The model under review builds one solid part; all positions refer to its coordinate system, in mm. A direction names the side the tool comes from. Give positions to 0.01 mm unless a question says otherwise; leave off trailing zeros. Write each loop counter-clockwise with the first axis right and the second up, starting at its lowest first coordinate (ties: lowest second). Pieces come first, ordered by that corner, then holes.
Autodesk Inventor part; units mm, degrees
ref_plane "Płaszczyzna konstrukcyjna1" through (0, -12, 0) normal (0, 0, -1) x (-1, 0, 0)
ref_plane "Płaszczyzna konstrukcyjna2" through (0, -10, -2.2657) normal (1, 0, 0) x (0, 0, -1)
ref_plane "YZ Plane" through (0, 0, 0) normal (1, 0, 0) x (0, 1, 0)
sketch "Szkic1" plane through (0, 0, 0) normal (0, 1, 0) x (-1, 0, 0)
  circle A0 centre (0, 0) radius 12.5
  circle A1 centre (0, 0) radius 10
  dimension "d0" = 20
  dimension "d2" = 25
extrude "Wyciągnięcie proste1" add sketch "Szkic1" along normal blind 5
ref_plane "Płaszczyzna konstrukcyjna1" through (0, -12, 0) normal (0, 0, -1) x (-1, 0, 0)
sketch "Szkic5" plane through (0, -12, 0) normal (0, 0, -1) x (-1, 0, 0)
  line L0 (12.5, 17) -> (-12.5, 17)
  line L1 (0, 17) -> (-12.5, 17)
  line L2 (-12.5, 17) -> (-12.5, 18.625)
  line L3 (-12.5, 18.625) -> (0, 18.625)
  line L4 (0, 18.625) -> (0, 17)
  line L5 (0, 18.625) -> (-9.5, 18.625)
  line L6 (-9.5, 18.625) -> (-9.5, 21.125)
  line L7 (-9.5, 21.125) -> (0, 21.125)
  line L8 (0, 21.125) -> (0, 18.625)
  line L9 (0, 21.125) -> (-12.5, 21.125)
  line L10 (-12.5, 21.125) -> (-12.5, 22.75)
  line L11 (-12.5, 22.75) -> (0, 22.75)
  line L12 (0, 22.75) -> (0, 21.125)
  line L13 (0, 22.75) -> (-9.5, 22.75)
  line L14 (-9.5, 22.75) -> (-9.5, 25.25)
  line L15 (-9.5, 25.25) -> (0, 25.25)
  line L16 (0, 25.25) -> (0, 22.75)
  line L17 (0, 25.25) -> (-12.5, 25.25)
  line L18 (-12.5, 25.25) -> (-12.5, 26.875)
  line L19 (-12.5, 26.875) -> (0, 26.875)
  line L20 (0, 26.875) -> (0, 25.25)
  line L21 (0, 26.875) -> (-9.5, 26.875)
  line L22 (-9.5, 26.875) -> (-9.5, 29.375)
  line L23 (-9.5, 29.375) -> (0, 29.375)
  line L24 (0, 29.375) -> (0, 26.875)
  line L25 (0, 29.375) -> (-12.5, 29.375)
  line L26 (-12.5, 29.375) -> (-12.5, 31)
  line L27 (-12.5, 31) -> (0, 31)
  line L28 (0, 31) -> (0, 29.375)
  line L29 (-12.5, 12) -> (-12.5, 17) construction
  line L30 (-12.5, 12) -> (-12.5, 17) construction
  line L31 (-12.5, 12) -> (12.5, 12) construction
  point P0 (0, 12)
  dimension "d13" = 2.5
  dimension "d17" = 19
  dimension "d18" = 3
revolve "Obrót1" add sketch "Szkic5" angle 360 about axis through (0, 10.75, 0) along (0, -1, 0)
sketch "Szkic7" plane through (0, 17.375, 0) normal (0, -1, 0) x (1, 0, 0)
  circle A0 centre (0, 0) radius 9.5
  circle A1 centre (0, 9.5) radius 1.65
  circle A2 centre (0, 0) radius 10
  circle A3 centre (0, 0) radius 9.5
  circle A4 centre (-9.5, 0) radius 1.65
  circle A5 centre (0, -9.5) radius 1.65
  circle A6 centre (9.5, 0) radius 1.65
  circle A7 centre (6.7175, -6.7175) radius 0.9
  circle A8 centre (6.7175, 6.7175) radius 0.9
  circle A9 centre (-6.7175, 6.7175) radius 0.9
  circle A10 centre (-6.7175, -6.7175) radius 0.9
  line L0 (6.7175, 6.7175) -> (0, 0) construction
  line L1 (0, 0) -> (-6.7175, 6.7175) construction
  circle A11 centre (0, 0) radius 12.5 construction
  line L2 (0, 0) -> (-6.7175, -6.7175) construction
  line L3 (0, 0) -> (6.7175, -6.7175) construction
  line L4 (17.5, 0) -> (-17.5, 0) construction
  dimension "d23" = 45
  dimension "d24" = 45
  dimension "d25" = 3.3
  dimension "d47" = 1.8
extrude "Wyciągnięcie proste6" cut sketch "Szkic7" along normal up to surface (10.75 mm away) contours A0 A6 | A0 A6 A2 | A8 A0 | A0 A8 A2 | A6 A2 | A7 A2 A0 | A0 A7 | A2 A8 | A7 A2 | A1 A0 | A0 A1 A2 | A5 A2 A0 | A0 A5 | A2 A1 | A5 A2 | A9 A0 | A0 A9 A2 | A10 A2 A0 | A0 A10 | A2 A9 | A10 A2 | A4 A0 | A0 A4 A2 | A2 A4
sketch "Szkic8" plane through (0, -12, 0) normal (0, 0, -1) x (-1, 0, 0)
  line L0 (6.0517, 25.25) -> (1.6438, 25.25)
  line L1 (-1.6438, 25.25) -> (-1.6438, 22.75)
  line L2 (1.6438, 25.25) -> (-1.6438, 25.25)
  line L3 (-1.6438, 25.25) -> (-1.6438, 22.75)
  line L4 (-1.6438, 22.75) -> (1.6438, 22.75)
  line L5 (1.6438, 22.75) -> (1.6438, 25.25)
  point P0 (0, 12)
  point P1 (1.65, 22.75)
extrude "Wyciągnięcie proste7" cut sketch "Szkic8" along normal through all both and the other way through all
sketch "Szkic9" plane through (0, 5, 0) normal (0, -1, 0) x (1, 0, 0)
  line L0 (0, 0) -> (-3.4352, 0)
  line L1 (-3.4352, 0) -> (-3.4352, -2.2657)
  line L2 (-3.4352, -2.2657) -> (0, -2.2657)
  line L3 (0, -2.2657) -> (0, 0)
  dimension "d30" = 3.4352
  dimension "d31" = 2.2658
extrude "Wyciągnięcie proste8" add sketch "Szkic9" along normal blind 15
ref_plane "Płaszczyzna konstrukcyjna2" through (0, -10, -2.2657) normal (1, 0, 0) x (0, 0, -1)
sketch "Szkic10" plane through (0, -10, 0) normal (0, -1, 0) x (1, 0, 0)
  line L0 (0, 0) -> (-3.4352, 0)
  line L1 (-3.4352, -2.2657) -> (0, -2.2657)
  line L2 (0, 0) -> (-3.4352, 0)
  line L3 (-3.4352, 0) -> (-3.4352, -2.2657)
  line L4 (-3.4352, -2.2657) -> (0, -2.2657)
  line L5 (0, -2.2657) -> (0, 0)
extrude "Wyciągnięcie proste9" cut sketch "Szkic10" against normal up to surface (15 mm away)
sketch "Szkic11" plane through (0, -10, -2.2657) normal (1, 0, 0) x (0, 0, -1)
  line L0 (-3.9095, 20.75) -> (-3.9095, 23.25)
  line L1 (-0.622, 20.75) -> (-0.622, 23.25)
  line L2 (-3.9095, 20.75) -> (-0.622, 20.75)
  line L3 (-0.622, 20.75) -> (-0.622, 23.25)
  line L4 (-0.622, 23.25) -> (-3.9095, 23.25)
  line L5 (-3.9095, 23.25) -> (-3.9095, 20.75)
  point P0 (-2.2657, 10)
extrude "Wyciągnięcie proste10" cut sketch "Szkic11" along normal through all both and the other way through all
sketch "Szkic12" plane through (0, 19, 0) normal (0, 1, 0) x (1, 0, 0)
  line L0 (0, 0) -> (4.6374, 4.6374) construction
  line L1 (0, 0) -> (6.5583, 0) construction
  line L2 (0, 0) -> (-4.6374, 4.6374) construction
  line L3 (0, 0) -> (-4.8503, -4.8503) construction
  line L4 (0, 0) -> (4.8503, -4.8503) construction
  point P0 (-4.6374, 4.6374)
  point P1 (4.6328, -4.7775)
  dimension "d39" = 6.5583
hole "Otwór1" at (4.6374, 19, -4.6374) at (-4.6374, 19, -4.6374) at (-4.8503, 19, 4.8503) at (4.6328, 19, 4.7775) direction (0, -1, 0) diameter 3.4 end through all countersink diameter 6.9 countersink angle 89.954
sketch "Szkic13" plane through (0, 5, 0) normal (0, -1, 0) x (1, 0, 0)
  circle A0 centre (0, 0) radius 2
  dimension "d48" = 4
extrude "Wyciągnięcie proste11" cut sketch "Szkic13" against normal blind 5
properties part number "Felga" material "Tworzywo sztuczne PMMA"
1) Insertion check: pin 1 (2 mm diameter, centred on x = -6, y = 9.5, fed in from -Z); pin 2 (7.5 mm diameter, centred on x = 4, z = 6, fed in from -Y); pin 3 (5 mm diameter, centred on x = 0, z = 0, fed in from -Y); pin 4 (4 mm diameter, centred on y = 12.5, z = 5.5, fed in from +X). Each pin has a flat end and moves straight along its axis. Give the tip position at first contact, or say it passes through.
2) Consider section D-D, the plane y = 8.5. Give the boundary of the cut face in (x, z).
3) Consider section C-C, the plane z = -10.75. Give the boundary of the cut face in (x, y) (3 decimals).
4) The part is to be moulded in two halves that separate along Y. For faces 1 (the conical face through (-3.627, 17.358, 3.517)), 2 (the flat face through (4, 9.125, -9)), 3 (the cylindrical face through (-3.34, 11.04, 5.63)), 4 (the cylindrical face through (0.89, 9.17, 8.11)), say which applies: +Y half, -Y half, draft (parallel to the pull), parting line (faces both ways), or undercut.
5) To check wall thickness, follow probe 1 along Y at (x, z) = (-7.25, 7.75) (3 decimals); probe 2 along Y at (x, z) = (-0.5, 5.75); probe 3 along Z at (x, y) = (0, 1.5). State the ranges of each line that lie inside material, in increasing order.
6) Tool access review of faces 5 (the cylindrical face through (-5.86, 12.08, 6.45)), 6 (the cylindrical face through (-8.64, 7.89, 3.95)), 7 (the cylindrical face through (3.95, 16.14, 8.64)): name each direction out of +Z, -Z, +X, -X, +Y, -Y from which nothing blocks a thin tool from reaching the whole face with its end or side.
Answer block:
1. pin 1: stops at z = -11.46
1. pin 2: stops at y = 0
1. pin 3: stops at y = 5
1. pin 4: stops at x = 11.96
2. outline: (-9.36, -1.64) arc R9.5 ccw to (-7.32, -6.05) arc R0.9 cw to (-6.05, -7.32) arc R9.5 ccw to (-1.64, -9.36) arc R1.65 cw to (1.64, -9.36) arc R9.5 ccw to (6.05, -7.32) arc R0.9 cw to (7.32, -6.05) arc R9.5 ccw to (9.36, -1.64) arc R1.65 cw to (9.36, 1.64) arc R9.5 ccw to (7.32, 6.05) arc R0.9 cw to (6.05, 7.32) arc R9.5 ccw to (1.64, 9.36) arc R1.65 cw to (-1.64, 9.36) arc R9.5 ccw to (-6.05, 7.32) arc R0.9 cw to (-7.32, 6.05) arc R9.5 ccw to (-9.36, 1.64) arc R1.65 cw to start; hole circle Ø3.4 at (-4.85, 4.85); hole circle Ø3.4 at (-4.64, -4.64); hole circle Ø4 at (0, 0); hole circle Ø3.4 at (4.63, 4.78); hole circle Ø3.4 at (4.64, -4.64)
3. outline: (-6.379, 0) - (6.379, 0) - (6.379, 6.625) - (-6.379, 6.625) - close; (-6.379, 9.125) - (-1.077, 9.125) - (-1.077, 10.75) - (-6.379, 10.75) - close; (-6.379, 13.25) - (-1.077, 13.25) - (-1.077, 14.875) - (-6.379, 14.875) - close; (-6.379, 17.375) - (6.379, 17.375) - (6.379, 19) - (-6.379, 19) - close; (1.077, 9.125) - (6.379, 9.125) - (6.379, 10.75) - (1.077, 10.75) - close; (1.077, 13.25) - (6.379, 13.25) - (6.379, 14.875) - (1.077, 14.875) - close
4. face 1: +Y half
4. face 2: undercut
4. face 3: draft
4. face 4: undercut
5. probe 1: y = 0 to 6.625, 9.125 to 10.75, 13.25 to 14.875, 17.375 to 19
5. probe 2: y = 5 to 10.75, 13.25 to 19
5. probe 3: z = -12.5 to -10, 10 to 12.5
6. face 5: none
6. face 6: +Z, -X
6. face 7: +Z, +X
